Input: dimensioned drawing with shaded views. Units: mm. Origin: part minimum x, y, z. A direction names the side the tool comes from. Round coordinates to 2 decimals unless told otherwise and drop trailing zeros. Loops run counter-clockwise (first coordinate to the right, second up) from the corner with the lowest first, then second, coordinate; pieces in that order, holes last. Notation, with made-up numbers: (34.25, 28.25) - (61.25, 28.25) arc R17 ccw to (61.25, 53.25) - close; hole circle Ø2 at (30, 84.25). An arc over 180 degrees is marked (long way). Answer as CSV lines item,"result".
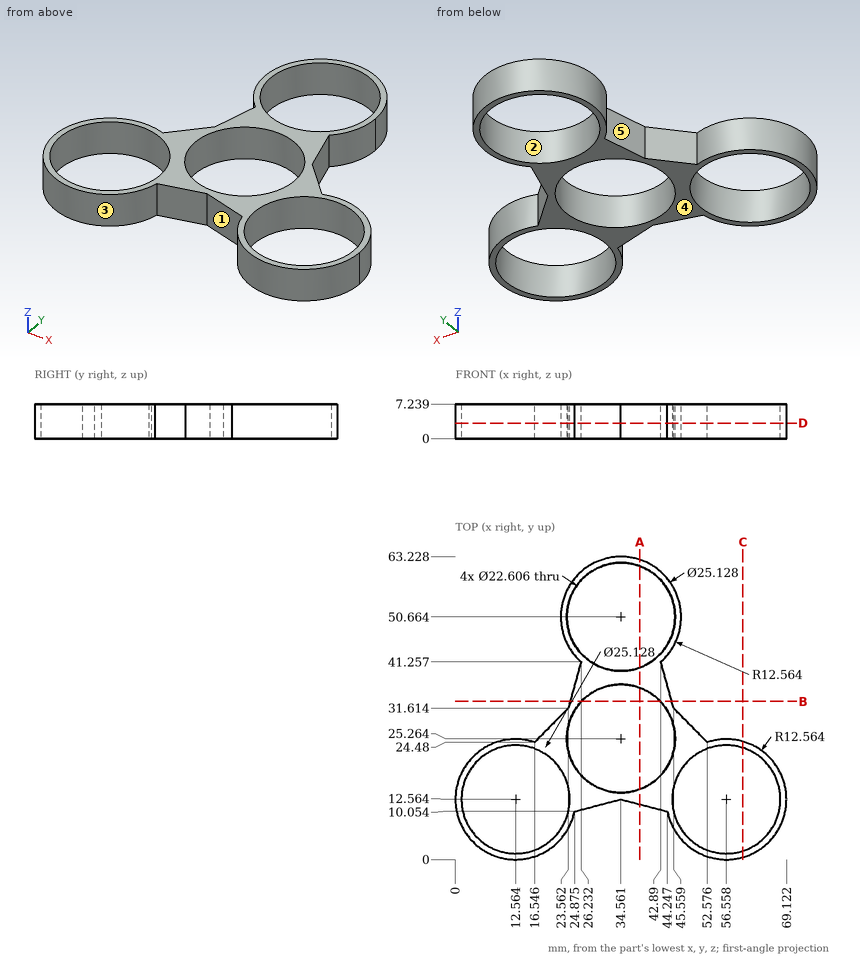
(1) Section A-A (x = 38.5). Output: boundary loops of the cut face in (y, z) (1 decimal).
Findings below:
outline,"(11.5, 0) - (14.7, 0) - (14.7, 7.2) - (11.5, 7.2) - close; (35.9, 0) - (40.1, 0) - (40.1, 7.2) - (35.9, 7.2) - close; (61.3, 0) - (62.6, 0) - (62.6, 7.2) - (61.3, 7.2) - close"
(2) Material intervals for line 1 along Y through (x, z) = (40, 6.25) (1 decimal); line 2 along X through (y, z) = (59, 4.25) (1 decimal); line 3 along X through (y, z) = (15, 0.5) (1 decimal), sorted ascending.
Findings below:
line 1,"11.2 to 15.4, 35.2 to 40.8, 60.6 to 62"
line 2,"25.2 to 26.9, 42.2 to 44"
line 3,"0.2 to 1.5, 23.6 to 29.8, 39.3 to 45.5, 67.6 to 68.9"
(3) Draft query along X for the marked faces 3, 4 and 5. Return one class per face: pulls with the +X half, pulls with the -X half, needs draft (parallel to the pull), parting line crosses it, or undercut.
Findings below:
face 3,"undercut"
face 4,"needs draft"
face 5,"pulls with the -X half"
(4) Section C-C (x = 60). Output: boundary loops of the cut face in (y, z).
Findings below:
outline,"(0.48, 0) - (1.8, 0) - (1.8, 7.24) - (0.48, 7.24) - close; (23.33, 0) - (24.65, 0) - (24.65, 7.24) - (23.33, 7.24) - close"
(5) Pin query (flat end, axial travel): P1, Ø13.5, axis at x = 34.56, y = 25.26, coming from the +Z side; P2, Ø1.5, axis at x = 8, z = 2.5, coming from the -Y side. Return the tip coordinate at first contact, or that it passes through.
Findings below:
P1,"through"
P2,"y = 0.59"
(6) Section B-B (y = 33). Output: boundary loops of the cut face in (x, z) (1 decimal).
Findings below:
outline,"(23.9, 0) - (26.3, 0) - (26.3, 7.2) - (23.9, 7.2) - close; (42.8, 0) - (45.2, 0) - (45.2, 7.2) - (42.8, 7.2) - close"
(7) Access query for the marked faces 1 and 2. Directions: +Z, -Z, +X, -X, +Y, -Y. A direction counts if a zero-diameter tool reaches every point of the face in a straight line with its end or side. Return the directions, or none.
Findings below:
face 1,"+Z, -Z, -Y"
face 2,"+Z, -Z"
(8) Section D-D (z = 3.25). Output: boundary loops of the cut face in (x, y) (1 decimal).
Findings below:
outline,"(16.5, 24.5) arc R12.6 ccw (long way) to (24.9, 10.1) - (34.6, 12.6) - (44.2, 10.1) arc R12.6 ccw (long way) to (52.6, 24.5) - (45.6, 31.6) - (42.9, 41.3) arc R12.6 ccw to (47.1, 50.7) arc R12.6 ccw (long way) to (26.2, 41.3) - (23.6, 31.6) - close; hole circle Ø22.6 at (12.6, 12.6); hole circle Ø22.6 at (34.6, 25.3); hole circle Ø22.6 at (34.6, 50.7); hole circle Ø22.6 at (56.6, 12.6)"
